Part print with two shaded views. Sizes in mm from the minimum x, y, z corner. A direction names the side the tool comes from. Give positions to 0.01 mm unless a question says otherwise; leave off trailing zeros. Write each loop counter-clockwise with the first axis right and the second up, starting at its lowest first coordinate (ties: lowest second). Pieces come first, ordered by that corner, then holes.
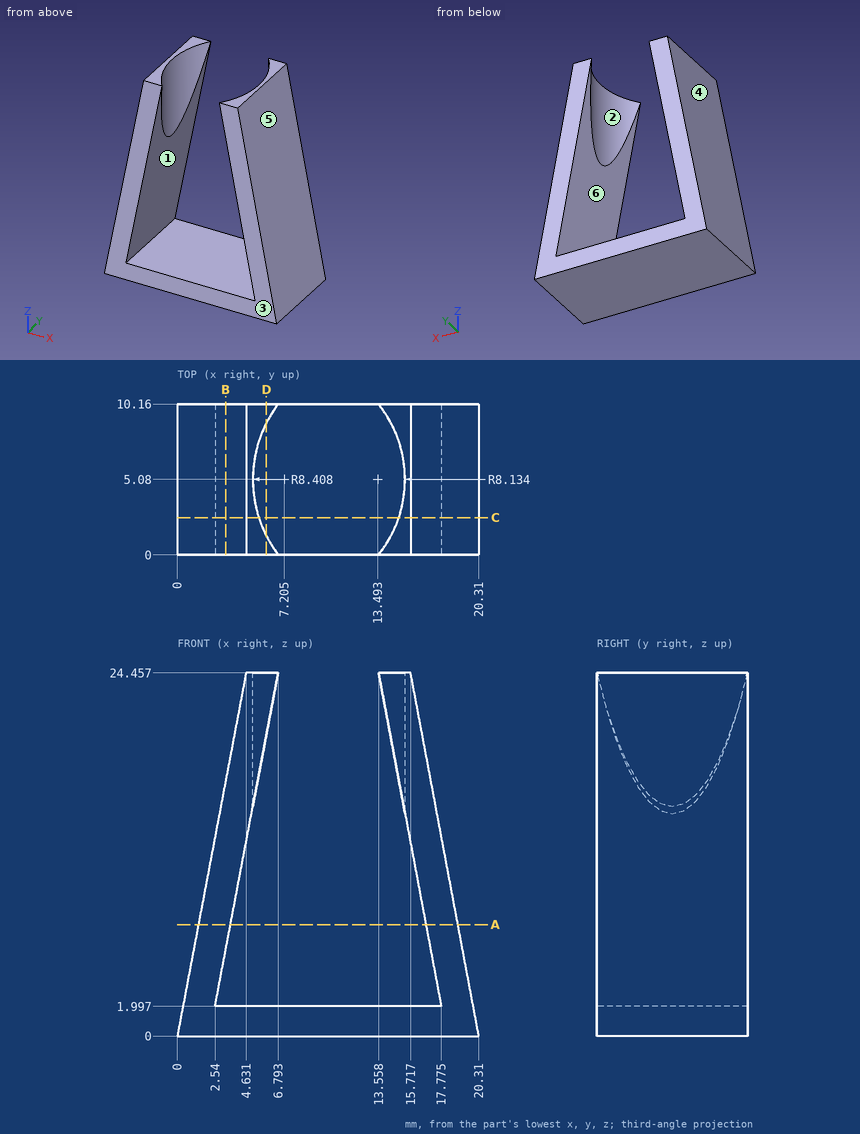
(1) Probe line 1 (Z direction, x = 11.5, y = 3.5); line 2 (X direction, y = 8.25, z = 6.75); line 3 (X direction, y = 1.5, z = 21.75) (1 decimal). List the from-to ranges inside material, lowest first.
(2) Saw through at A-A, the plane z = 7.5. List the corners of the cut face in (x, y).
(3) Saw through at B-B, the plane x = 3.25. List the corners of the cut face in (y, z), plus the area to 3 significant figures.
(4) Saw through at C-C, the plane y = 2.5. List the corners of the cut face in (x, z) (1 decimal).
(5) Drop flat-ended pins along their axis: pin 1 (1 mm diameter, centred on y = 9, z = 10.5, fed in from +X); pin 2 (1.5 mm diameter, centred on x = 8.5, y = 3, fed in from +Z); pin 3 (3 mm diameter, centred on y = 7.5, z = 21, fed in from +X). Give the stop position or say it passes through.
(6) Saw through at D-D, the plane x = 6. List the corners of the cut face in (y, z) (1 decimal).
(7) Mould opens along X. For the marked faces 4, 5 and 6 say: +X half, -X half, draft (parallel to the pull), parting line (faces both ways), or undercut.
(8) 3-axis set-ups, long thin cutter, end or side, ignore diameter. For the marked faces 1, 2 and 3: which of +Z, -Z, +X, -X, +Y, -Y reach the whole face in a straight line?
Computed values:
1. line 1: z = 0 to 2
1. line 2: x = 1.28 to 3.44, 16.88 to 19.04
1. line 3: x = 4.1 to 5.9, 14.5 to 16.2
2. outline: (1.42, 0) - (3.58, 0) - (3.58, 10.16) - (1.42, 10.16) - close; (16.74, 0) - (18.9, 0) - (18.9, 10.16) - (16.74, 10.16) - close
3. outline: (0, 0) - (10.16, 0) - (10.16, 2) - (0, 2) - close; (0, 5.75) - (10.16, 5.75) - (10.16, 17.16) - (0, 17.16) - close
3. area: 136 mm2
4. outline: (0, 0) - (20.3, 0) - (15.7, 24.5) - (14.9, 24.5) - (14.9, 17.2) - (17.8, 2) - (2.5, 2) - (5.5, 17.6) - (5.5, 24.5) - (4.6, 24.5) - close
5. pin 1: stops at x = 18.43
5. pin 2: stops at z = 2
5. pin 3: stops at x = 16.65
6. outline: (0, 0) - (10.2, 0) - (10.2, 2) - (0, 2) - close; (0, 20.3) - (1.3, 20.3) - (1.3, 24.5) - (0, 24.5) - close; (8.9, 20.3) - (10.2, 20.3) - (10.2, 24.5) - (8.9, 24.5) - close
7. face 4: -X half
7. face 5: +X half
7. face 6: undercut
8. face 1: +Y, -Y
8. face 2: +Z
8. face 3: +Z, -Z, +X, -X, -Y
